Could you check a few things on this model? Use its own coordinates, in mm. Face numbers are marked on the shaded views. Give positions to 0.01 mm unless a question says otherwise; leave off trailing zeros. Order: outer loops, then holes, each group sorted by start corner. A loop starts at its lowest first (then second) coordinate and runs counter-clockwise, first axis right, second up.
(1) Imagine slicing it at B-B, the plane z = 41. State how many separate pieces and enclosed holes the cut face has, then the cut area to 3 significant figures.
(2) If I drill on probe 1 along Y at (x, z) = (135, 19); probe 2 along Y at (x, z) = (103, 10.5); probe 3 along Z at (x, y) = (97, 15.5), over which ranges is the centre line in solid material (lowest first)?
(3) Will this pin go through, and if not, where does the flat tip stop? pin 1 (10.5 mm diameter, centred on x = 58.5, y = 84, fed in from +Z).
(4) Imagine slicing it at A-A, the plane x = 12.5. Write out the boundary of the cut face in (y, z).
(5) If we mould it in two halves opening along Y, with no side actions, what happens to the marked faces 1, 2 and 3? For each: released by +Y, released by -Y, zero draft, split by the parting line, or undercut.
(6) Imagine slicing it at C-C, the plane x = 68. Write out the boundary of the cut face in (y, z), then the cut area to 3 significant figures.
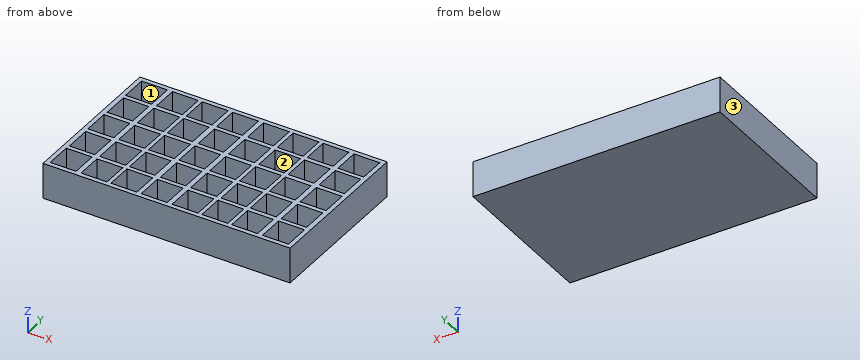
from build123d import *

# Parameters (mm, degrees)
SKETCH1_W           = 334
SKETCH1_H           = 211
SKETCH1_W_2         = 34.277630703
SKETCH1_H_2         = 35.361184648
SKETCH1_W_3         = 35
SKETCH1_H_3         = 35
SKETCH1_H_4         = 34.638815352
BOSS_EXTRUDE1_DEPTH = 45
SKETCH2_W           = 334
SKETCH2_H           = 211
BOSS_EXTRUDE2_DEPTH = 3


with BuildPart() as part:
    # Sketch1 → Boss-Extrude1 (new body)
    with BuildSketch(Plane.XY):
        Rectangle(SKETCH1_W, SKETCH1_H)
        with Locations((143.138815351, 41.180592324)):
            Rectangle(SKETCH1_W_2, SKETCH1_H_2, mode=Mode.SUBTRACT)
        with Locations((143.5, 82)):
            Rectangle(SKETCH1_W_3, SKETCH1_H_3, mode=Mode.SUBTRACT)
        with Locations((61.5, 82)):
            Rectangle(SKETCH1_W_3, SKETCH1_H_3, mode=Mode.SUBTRACT)
        with Locations((61.861184649, 41.180592324)):
            Rectangle(SKETCH1_W_2, SKETCH1_H_2, mode=Mode.SUBTRACT)
        with Locations((101.777630703, 82.180592324)):
            Rectangle(SKETCH1_W_3, SKETCH1_H_4, mode=Mode.SUBTRACT)
        with Locations((101.777630703, 41.180592324)):
            Rectangle(SKETCH1_W_3, SKETCH1_H_2, mode=Mode.SUBTRACT)
        with Locations((143.138815351, -41.180592324)):
            Rectangle(SKETCH1_W_2, SKETCH1_H_2, mode=Mode.SUBTRACT)
        with Locations((101.777630703, -41.180592324)):
            Rectangle(SKETCH1_W_3, SKETCH1_H_2, mode=Mode.SUBTRACT)
        with Locations((61.861184649, -41.180592324)):
            Rectangle(SKETCH1_W_2, SKETCH1_H_2, mode=Mode.SUBTRACT)
        with Locations((61.5, -82)):
            Rectangle(SKETCH1_W_3, SKETCH1_H_3, mode=Mode.SUBTRACT)
        with Locations((101.777630703, -82.180592324)):
            Rectangle(SKETCH1_W_3, SKETCH1_H_4, mode=Mode.SUBTRACT)
        with Locations((143.5, -82)):
            Rectangle(SKETCH1_W_3, SKETCH1_H_3, mode=Mode.SUBTRACT)
        with Locations((-143.5, -82)):
            Rectangle(SKETCH1_W_3, SKETCH1_H_3, mode=Mode.SUBTRACT)
        with Locations((-101.777630703, -82.180592324)):
            Rectangle(SKETCH1_W_3, SKETCH1_H_4, mode=Mode.SUBTRACT)
        with Locations((-61.5, -82)):
            Rectangle(SKETCH1_W_3, SKETCH1_H_3, mode=Mode.SUBTRACT)
        with Locations((-61.861184649, -41.180592324)):
            Rectangle(SKETCH1_W_2, SKETCH1_H_2, mode=Mode.SUBTRACT)
        with Locations((-101.777630703, -41.180592324)):
            Rectangle(SKETCH1_W_3, SKETCH1_H_2, mode=Mode.SUBTRACT)
        with Locations((-143.138815351, -41.180592324)):
            Rectangle(SKETCH1_W_2, SKETCH1_H_2, mode=Mode.SUBTRACT)
        with Locations((-143.138815351, 41.180592324)):
            Rectangle(SKETCH1_W_2, SKETCH1_H_2, mode=Mode.SUBTRACT)
        with Locations((-101.777630703, 41.180592324)):
            Rectangle(SKETCH1_W_3, SKETCH1_H_2, mode=Mode.SUBTRACT)
        with Locations((-61.861184649, 41.180592324)):
            Rectangle(SKETCH1_W_2, SKETCH1_H_2, mode=Mode.SUBTRACT)
        with Locations((-61.5, 82)):
            Rectangle(SKETCH1_W_3, SKETCH1_H_3, mode=Mode.SUBTRACT)
        with Locations((-101.777630703, 82.180592324)):
            Rectangle(SKETCH1_W_3, SKETCH1_H_4, mode=Mode.SUBTRACT)
        with Locations((-143.5, 82)):
            Rectangle(SKETCH1_W_3, SKETCH1_H_3, mode=Mode.SUBTRACT)
        with Locations((61.5, 0)):
            Rectangle(SKETCH1_W_3, SKETCH1_H_3, mode=Mode.SUBTRACT)
        with Locations((101.777630703, -0.180592324)):
            Rectangle(SKETCH1_W_3, SKETCH1_H_4, mode=Mode.SUBTRACT)
        with Locations((143.5, 0)):
            Rectangle(SKETCH1_W_3, SKETCH1_H_3, mode=Mode.SUBTRACT)
        with Locations((-143.5, 0)):
            Rectangle(SKETCH1_W_3, SKETCH1_H_3, mode=Mode.SUBTRACT)
        with Locations((-101.777630703, -0.180592324)):
            Rectangle(SKETCH1_W_3, SKETCH1_H_4, mode=Mode.SUBTRACT)
        with Locations((-61.5, 0)):
            Rectangle(SKETCH1_W_3, SKETCH1_H_3, mode=Mode.SUBTRACT)
        with Locations((-20.5, 82)):
            Rectangle(SKETCH1_W_3, SKETCH1_H_3, mode=Mode.SUBTRACT)
        with Locations((-20.138815351, 41.180592324)):
            Rectangle(SKETCH1_W_2, SKETCH1_H_2, mode=Mode.SUBTRACT)
        with Locations((-20.5, 0)):
            Rectangle(SKETCH1_W_3, SKETCH1_H_3, mode=Mode.SUBTRACT)
        with Locations((-20.138815351, -41.180592324)):
            Rectangle(SKETCH1_W_2, SKETCH1_H_2, mode=Mode.SUBTRACT)
        with Locations((-20.5, -82)):
            Rectangle(SKETCH1_W_3, SKETCH1_H_3, mode=Mode.SUBTRACT)
        with Locations((21.222369297, -82.180592324)):
            Rectangle(SKETCH1_W_3, SKETCH1_H_4, mode=Mode.SUBTRACT)
        with Locations((21.222369297, -41.180592324)):
            Rectangle(SKETCH1_W_3, SKETCH1_H_2, mode=Mode.SUBTRACT)
        with Locations((21.222369297, -0.180592324)):
            Rectangle(SKETCH1_W_3, SKETCH1_H_4, mode=Mode.SUBTRACT)
        with Locations((21.222369297, 41.180592324)):
            Rectangle(SKETCH1_W_3, SKETCH1_H_2, mode=Mode.SUBTRACT)
        with Locations((21.222369297, 82.180592324)):
            Rectangle(SKETCH1_W_3, SKETCH1_H_4, mode=Mode.SUBTRACT)
    extrude(amount=BOSS_EXTRUDE1_DEPTH)

    # Sketch2 → Boss-Extrude2 (add)
    with BuildSketch(Plane(origin=(0, 0, 0), x_dir=(-1, 0, 0), z_dir=(0, 0, -1))):
        Rectangle(SKETCH2_W, SKETCH2_H)
    extrude(amount=BOSS_EXTRUDE2_DEPTH)


solid = part.part
Answer block:
1. separate pieces: 1
1. enclosed holes: 40
1. area: 21,600 mm2
2. probe 1: y = -105.5 to -99.5, -64.5 to -58.86, -23.5 to -17.5, 17.5 to 23.5, 58.86 to 64.5, 99.5 to 105.5
2. probe 2: y = -105.5 to -99.5, -64.86 to -58.86, -23.5 to -17.5, 17.14 to 23.5, 58.86 to 64.86, 99.5 to 105.5
2. probe 3: z = -3 to 0
3. pin 1: stops at z = 0
4. outline: (-105.5, -3) - (105.5, -3) - (105.5, 45) - (99.5, 45) - (99.5, 0) - (64.86, 0) - (64.86, 45) - (58.86, 45) - (58.86, 0) - (23.5, 0) - (23.5, 45) - (17.14, 45) - (17.14, 0) - (-17.5, 0) - (-17.5, 45) - (-23.5, 45) - (-23.5, 0) - (-58.86, 0) - (-58.86, 45) - (-64.86, 45) - (-64.86, 0) - (-99.5, 0) - (-99.5, 45) - (-105.5, 45) - close
5. face 1: undercut
5. face 2: undercut
5. face 3: zero draft
6. outline: (-105.5, -3) - (105.5, -3) - (105.5, 45) - (99.5, 45) - (99.5, 0) - (64.5, 0) - (64.5, 45) - (58.86, 45) - (58.86, 0) - (23.5, 0) - (23.5, 45) - (17.5, 45) - (17.5, 0) - (-17.5, 0) - (-17.5, 45) - (-23.5, 45) - (-23.5, 0) - (-58.86, 0) - (-58.86, 45) - (-64.5, 45) - (-64.5, 0) - (-99.5, 0) - (-99.5, 45) - (-105.5, 45) - close
6. area: 2,220 mm2
